Autodesk Inventor part; units mm, degrees
ref_plane "YZ Plane" through (0, 0, 0) normal (1, 0, 0) x (0, 1, 0)
ref_plane "XZ Plane" through (0, 0, 0) normal (0, 1, 0) x (-1, 0, 0)
ref_plane "XY Plane" through (0, 0, 0) normal (0, 0, 1) x (1, 0, 0)
sketch "Board outline" plane through (0, 0, 0) normal (0, 0, 1) x (1, 0, 0)
  line L0 (-95, 95) -> (95, 95)
  line L1 (95, 95) -> (95, -95)
  line L2 (95, -95) -> (-95, -95)
  line L3 (-95, -95) -> (-95, 95)
  circle A0 centre (92, 92) radius 12.5002
  circle A1 centre (-92, 92) radius 12.5002
  circle A2 centre (92, -92) radius 12.5002
  circle A3 centre (-92, -92) radius 12.5002
  point P0 (-79.8652, -95)
  point P1 (79.8652, -95)
  point P2 (95, -79.8651)
  point P3 (95, 79.8651)
  point P4 (79.8652, 95)
  point P5 (-79.8652, 95)
  point P6 (-95, 79.8651)
  point P7 (-95, -79.8651)
extrude "Extrusion1" add sketch "Board outline" along normal blind 3
sketch "Level 2-3 #6 standoff holes" plane through (0, 0, 3) normal (0, 0, 1) x (1, 0, 0)
  circle A0 centre (92, 92) radius 1.8984
  circle A1 centre (-92, -92) radius 1.8984
  circle A2 centre (-92, 92) radius 1.8984
  circle A3 centre (92, -92) radius 1.8984
sketch "B210 countersink holes" plane through (0, 0, 0) normal (0, 0, 1) x (1, 0, 0)
  circle A0 centre (46.8, 60) radius 1.4998
  circle A1 centre (-46.8, 60) radius 1.4998
  circle A2 centre (46.8, -60) radius 1.4998
  circle A3 centre (-46.8, -60) radius 1.4998
sketch "OpenUPS mount holes" plane through (0, 0, 3) normal (0, 0, 1) x (1, 0, 0)
  circle A0 centre (85.86, 28.3) radius 1.5002
  circle A1 centre (85.86, -48.3) radius 1.5002
  circle A2 centre (24.14, 28.3) radius 1.5002
  circle A3 centre (24.14, -48.3) radius 1.5002
hole "Hole2" at (46.8, 60, 0) at (-46.8, 60, 0) at (-46.8, -60, 0) at (46.8, -60, 0) direction (0, 0, 1) diameter 2.459 end through all countersink diameter 6 countersink angle 90
hole "Hole3" at (24.14, 28.3, 3) at (85.86, 28.3, 3) at (85.86, -48.3, 3) at (24.14, -48.3, 3) direction (0, 0, -1) diameter 2.459 end through all countersink diameter 6 countersink angle 90
sketch "Level 1-2 #6 standoff holes" plane through (0, 0, 3) normal (0, 0, 1) x (1, 0, 0)
  circle A0 centre (80, 80) radius 1.8983
  circle A1 centre (-80, 80) radius 1.8983
  circle A2 centre (80, -80) radius 1.8983
  circle A3 centre (-80, -80) radius 1.8983
sketch "Level 1 M3 standoff holes" plane through (0, 0, 3) normal (0, 0, 1) x (1, 0, 0)
  circle A0 centre (70, 80) radius 1.4998
  circle A1 centre (-70, 80) radius 1.4998
  circle A2 centre (-70, -80) radius 1.4998
  circle A3 centre (70, -80) radius 1.4998
hole "Hole4" at (-70, 80, 3) at (70, 80, 3) at (70, -80, 3) at (-70, -80, 3) direction (0, 0, -1) diameter 3.4 end through all
hole "Hole5" at (-80, 80, 3) at (80, 80, 3) at (80, -80, 3) at (-80, -80, 3) direction (0, 0, -1) diameter 3.797 end through all
hole "Hole6" at (-92, -92, 3) at (92, -92, 3) at (92, 92, 3) at (-92, 92, 3) direction (0, 0, -1) diameter 3.797 end through all
sketch "Cable cutouts" plane through (0, 0, 3) normal (0, 0, 1) x (1, 0, 0)
  line L0 (-76.0002, 58.0001) -> (-75.9998, 58.0001)
  line L1 (-75.9998, 5.9999) -> (-76.0002, 5.9999)
  arc A0 (-81.5002, -8.5001) -> (-76.0002, -14.0001) centre (-76.0002, -8.5001) ccw
  arc A1 (-70.4998, 32.5001) -> (-75.9998, 38.0001) centre (-75.9998, 32.5001) ccw
  arc A2 (-76.0002, 38.0001) -> (-81.5002, 32.5001) centre (-76.0002, 32.5001) ccw
  line L2 (-81.5002, -8.5001) -> (-81.5002, 32.5001)
  line L3 (-75.9998, -14.0001) -> (-76.0002, -14.0001)
  line L4 (-70.4998, 32.5001) -> (-70.4998, -8.5001)
  line L5 (-76.0002, 38.0001) -> (-75.9998, 38.0001)
  arc A3 (-75.9998, -14.0001) -> (-70.4998, -8.5001) centre (-75.9998, -8.5001) ccw
  line L6 (66.8002, 5.2998) -> (66.7998, 5.2998)
  line L7 (71.7998, 0.2998) -> (71.7998, -55.6998)
  line L8 (66.7998, -60.6998) -> (66.8002, -60.6998)
  line L9 (61.8002, -55.6998) -> (61.8002, 0.2998)
  arc A4 (66.8002, 5.2998) -> (61.8002, 0.2998) centre (66.8002, 0.2998) ccw
  arc A5 (71.7998, 0.2998) -> (66.7998, 5.2998) centre (66.7998, 0.2998) ccw
  arc A6 (61.8002, -55.6998) -> (66.8002, -60.6998) centre (66.8002, -55.6998) ccw
  arc A7 (66.7998, -60.6998) -> (71.7998, -55.6998) centre (66.7998, -55.6998) ccw
  point P0 (66.8, -27.7)
  point P1 (66.8, 5.2998)
  dimension "d58" = 5.5
  dimension "d60" = 5
extrude "Extrusion2" cut sketch "Cable cutouts" against normal blind 3
sketch "5v Pololu regulator mount holes" plane through (0, 0, 3) normal (0, 0, 1) x (1, 0, 0)
  circle A0 centre (-72.5, -22.25) radius 1.2501
  circle A1 centre (-87.5, -22.25) radius 1.2501
  circle A2 centre (-72.5, -57.75) radius 1.2501
  circle A3 centre (-87.5, -57.75) radius 1.2501
hole "Hole7" at (-87.5, -22.25, 3) at (-72.5, -22.25, 3) at (-72.5, -57.75, 3) at (-87.5, -57.75, 3) direction (0, 0, -1) diameter 2.9 end through all
properties part number "payload_bay_b210_inventor" material "ABS Plastic"
Input: part model. Units: mm. Frame: model coordinates. Give positions to 0.01 mm unless a question says otherwise; leave off trailing zeros. Order: outer loops, then holes, each group sorted by start corner. A loop starts at its lowest first (then second) coordinate and runs counter-clockwise, first axis right, second up. Notation, with made-up numbers: (71.5, 86) - (110.5, 86) arc R26 cw to (110.5, 114) - close; hole circle Ø2 at (13.5, 8.5). An arc over 180 degrees is marked (long way). Use a Markdown table: item, result.
(1) Draft query along X for faces 1 (the flat face through (-1, 1, 3)), 2 (the conical face through (23.63, -49.54, 1.34)). Return one class per face: released by +X, released by -X, zero draft, split by the parting line, or undercut.
Computed values:
| item | result |
|---|---|
| face 1 | zero draft |
| face 2 | undercut |
(2) Line query: line 1 (X direction, y = -3, z = 1.4); line 2 (X direction, y = -22.25, z = 1.5); line 3 (X direction, y = 60, z = 2.7). Output: solid intervals per line, ascending. Write a range as from..to.
Computed values:
| item | result |
|---|---|
| line 1 | x = -95..-81.5, -70.5..61.8, 71.8..95 |
| line 2 | x = -95..-88.95, -86.05..-73.95, -71.05..61.8, 71.8..95 |
| line 3 | x = -95..-48.03, -45.57..45.57, 48.03..95 |
(3) Section query B-B (x = 34). Output: boundary loops of the cut face in (y, z), then the cut area to 3 significant figures.
Computed values:
| item | result |
|---|---|
| outline | (-95, 0) - (95, 0) - (95, 3) - (-95, 3) - close |
| area | 570 mm2 |
(4) Section query A-A (z = 0.45). State how many separate pieces and enclosed holes the cut face has, then the cut area to 3 significant figures.
Computed values:
| item | result |
|---|---|
| separate pieces | 1 |
| enclosed holes | 26 |
| area | 35,800 mm2 |
(5) Pin query (flat end, axial travel): pin 1 (3.5 mm diameter, centred on x = -80, y = -80, fed in from +Z); pin 2 (1.5 mm diameter, centred on y = -0.5, z = 1.5, fed in from -X); pin 3 (1.5 mm diameter, centred on x = 46, z = 1.5, fed in from +Y); pin 4 (1 mm diameter, centred on x = 6, z = 2.5, fed in from -Y). Return the tip coordinate at first contact, or that it passes through.
Computed values:
| item | result |
|---|---|
| pin 1 | passes through |
| pin 2 | stops at x = -95 |
| pin 3 | stops at y = 95 |
| pin 4 | stops at y = -95 |
